```python
from build123d import *

# Parameters (mm, degrees)
SKETCH1_W           = 62.4
SKETCH1_H           = 28
BOSS_EXTRUDE2_DEPTH = 7
SKETCH3_R           = 12.25
CUT_EXTRUDE2_DEPTH  = 6
CUT_EXTRUDE3_REACH  = 53.513
SKETCH4_W           = 18.2
SKETCH4_H           = 11
FILLET1_R           = 10
FILLET2_R           = 10
SKETCH5_W           = 3.5
SKETCH5_H           = 17
BOSS_EXTRUDE3_DEPTH = 20
SKETCH6_R           = 1.6
CUT_EXTRUDE4_DEPTH  = 72.38585011


with BuildPart() as part:
    # Sketch1 → Boss-Extrude2 (new body)
    with BuildSketch(Plane.XY):
        with Locations((14.966835682, -7.752691308)):
            Rectangle(SKETCH1_W, SKETCH1_H)
    extrude(amount=BOSS_EXTRUDE2_DEPTH)

    # Sketch3 → Cut-Extrude2 (cut)
    with BuildSketch(Plane.XY.offset(7)):
        with Locations((14.966835682, -6.752691308)):
            Circle(SKETCH3_R)
    extrude(amount=-CUT_EXTRUDE2_DEPTH, mode=Mode.SUBTRACT)

    # Sketch4 → Cut-Extrude3 (cut, up to next)
    with BuildSketch(Plane.XY.offset(7), mode=Mode.PRIVATE) as cut_extrude3_sk1:
        with Locations((-7.133164318, 0.747308692)):
            Rectangle(SKETCH4_W, SKETCH4_H)
    cut_extrude3_tool1 = extrude(cut_extrude3_sk1.sketch, amount=-CUT_EXTRUDE3_REACH, mode=Mode.PRIVATE) & part.part
    # Sketch4 → Cut-Extrude3 (cut, up to next)
    with BuildSketch(Plane.XY.offset(7), mode=Mode.PRIVATE) as cut_extrude3_sk2:
        with Locations((37.066835682, 0.747308692)):
            Rectangle(SKETCH4_W, SKETCH4_H)
    cut_extrude3_tool2 = extrude(cut_extrude3_sk2.sketch, amount=-CUT_EXTRUDE3_REACH, mode=Mode.PRIVATE) & part.part
    add(cut_extrude3_tool1.solids().sort_by_distance((-7.133164, 0.747309, 7))[0], mode=Mode.SUBTRACT)
    add(cut_extrude3_tool2.solids().sort_by_distance((37.066836, 0.747309, 7))[0], mode=Mode.SUBTRACT)

    # Fillet1
    fillet1_edges = [part.edges().sort_by_distance(p)[0] for p in [
        (1.966835682, -4.752691308, 3.5),
        (27.966835682, -4.752691308, 3.5),
    ]]
    fillet(fillet1_edges, radius=FILLET1_R)

    # Fillet2
    fillet2_edges = [part.edges().sort_by_distance(p)[0] for p in [
        (27.966835682, 6.247308692, 3.5),
        (1.966835682, 6.247308692, 3.5),
    ]]
    fillet(fillet2_edges, radius=FILLET2_R)

    # Sketch5 → Boss-Extrude3 (add)
    with BuildSketch(Plane.XY.offset(7)):
        with Locations((-14.483164318, -13.252691308)):
            Rectangle(SKETCH5_W, SKETCH5_H)
        with Locations((44.416835682, -13.252691308)):
            Rectangle(SKETCH5_W, SKETCH5_H)
    extrude(amount=BOSS_EXTRUDE3_DEPTH)

    # Sketch6 → Cut-Extrude4 (cut, through all)
    with BuildSketch(Plane.ZY.offset(16.233164318)):
        with Locations(Location((21, -10.252691308, 0), (0, 0, 270))):
            Circle(SKETCH6_R)
    extrude(amount=-CUT_EXTRUDE4_DEPTH, mode=Mode.SUBTRACT)


solid = part.part
```
Read the model definition and answer for the solid it produces. Units are mm, in the model's axes. A direction names the side the tool comes from. Give positions to 0.01 mm unless a question says otherwise; leave off trailing zeros. Write each loop counter-clockwise with the first axis right and the second up, starting at its lowest first coordinate (ties: lowest second). Pieces come first, ordered by that corner, then holes. Notation, with made-up numbers: (27.25, 53.25) -> (53.25, 53.25) arc R18 ccw to (53.25, 65.25) -> close; hole circle Ø8 at (6, 58). An arc over 180 degrees is marked (long way). Answer in a Markdown table with one row per item.
1) Section C-C on y = -1.5 is taken. Give the vertices of the cut face in (x, z), plus the area to 3 significant figures.
Results list:
| item | result |
|---|---|
| outline | (-0.65, 0) -> (30.59, 0) -> (30.59, 7) -> (26.03, 7) -> (26.03, 1) -> (3.9, 1) -> (3.9, 7) -> (-0.65, 7) -> close |
| area | 85.9 mm^2 |
2) Each of these flat-tipped pins is pushed along its axis until it touches: pin 1 Ø3 at (x, y) = (4, 0) entering from +Z; pin 2 Ø14 at (x, y) = (12, -4) entering from +Z; pin 3 Ø10 at (x, z) = (4.5, 3) entering from +Y. Where does it stop, or does it pass through?
Results list:
| item | result |
|---|---|
| pin 1 | z = 7 |
| pin 2 | z = 1 |
| pin 3 | y = 6.24 |
3) Section D-D on y = -17.25 is taken. Give the vertices of the cut face in (x, z), plus the area to 3 significant figures.
Results list:
| item | result |
|---|---|
| outline | (-16.23, 0) -> (46.17, 0) -> (46.17, 27) -> (42.67, 27) -> (42.67, 7) -> (21.28, 7) -> (21.28, 1) -> (8.65, 1) -> (8.65, 7) -> (-12.73, 7) -> (-12.73, 27) -> (-16.23, 27) -> close |
| area | 501 mm^2 |
4) Determine the mould class of faces 1 (the flat face through (44, -13, 27)), 2 (the flat face through (15, -7, 1)), 3 (the cylindrical face through (44.392, -10.044, 22.586)), 4 (the cylindrical face through (32.66, -3.23, 3.45)) for opening direction Y: released by +Y, released by -Y, zero draft, split by the parting line, or undercut.
Results list:
| item | result |
|---|---|
| face 1 | zero draft |
| face 2 | undercut |
| face 3 | undercut |
| face 4 | released by +Y |
5) Section B-B on z = 10.25 is taken. Give the vertices of the cut face in (x, y), plus the area to 3 significant figures.
Results list:
| item | result |
|---|---|
| outline | (-16.23, -21.75) -> (-12.73, -21.75) -> (-12.73, -4.75) -> (-16.23, -4.75) -> close; (42.67, -21.75) -> (46.17, -21.75) -> (46.17, -4.75) -> (42.67, -4.75) -> close |
| area | 119 mm^2 |
6) Straight lines are drawn through the part: line 1 (X direction, y = -6.5, z = 20); line 2 (Z direction, x = -3.5, y = -5.5); line 3 (Z direction, x = 18.5, y = -12.75). For each, find the intervals that lie inside material, in ascending order. Write a range as [from, to].
Results list:
| item | result |
|---|---|
| line 1 | [-16.23, -12.73], [42.67, 46.17] |
| line 2 | [0, 7] |
| line 3 | [0, 1] |
7) Section A-A on z = 21 is taken. Give the vertices of the cut face in (x, y).
Results list:
| item | result |
|---|---|
| outline | (-16.23, -21.75) -> (-12.73, -21.75) -> (-12.73, -11.85) -> (-16.23, -11.85) -> close; (-16.23, -8.65) -> (-12.73, -8.65) -> (-12.73, -4.75) -> (-16.23, -4.75) -> close; (42.67, -21.75) -> (46.17, -21.75) -> (46.17, -11.85) -> (42.67, -11.85) -> close; (42.67, -8.65) -> (46.17, -8.65) -> (46.17, -4.75) -> (42.67, -4.75) -> close |
8) A tool of negligible diameter and unlimited length cuts with its end or side. For faces 5 (the flat face through (-12.733, -13, 17)), 6 (the cylindrical face through (26.65, -3.07, 4.04)), 7 (the flat face through (44, -4.753, 11)), 8 (the flat face through (-14, -4.753, 10)), from which of +Z, -Z, +X, -X, +Y, -Y can it reach the whole face along a straight path? Write none if from no direction.
Results list:
| item | result |
|---|---|
| face 5 | +Z, +Y, -Y |
| face 6 | +Z |
| face 7 | +Z, -Z, +X, +Y |
| face 8 | +Z, -Z, -X, +Y |
